from build123d import *

# Parameters (mm, degrees)
F0_R     = 11.25
F0_R_2   = 4.25
F1_DEPTH = 5.5
F2_SIZE2 = 6.25
F2_SIZE  = 1
F0_R_3   = 14
F3_DEPTH = 6
F4_SIZE  = 0.4


with BuildPart() as f1:
    # F0 (on Top) → F1 (new body)
    with BuildSketch(Plane.XY):
        Circle(F0_R)
        Circle(F0_R_2, mode=Mode.SUBTRACT)
    extrude(amount=F1_DEPTH)

    # F2
    f2_edges = [f1.edges().sort_by_distance(p)[0] for p in [
        (-4.25, 0, 5.5),
    ]]
    chamfer(f2_edges, length=F2_SIZE, length2=F2_SIZE2)

    # F0 (on Top) → F3 (join)
    with BuildSketch(Plane.XY):
        Circle(F0_R_3)
        Circle(F0_R, mode=Mode.SUBTRACT)
    extrude(amount=F3_DEPTH)

    # F4
    f4_edges = [f1.edges().sort_by_distance(p)[0] for p in [
        (-11.25, 0, 6),
    ]]
    chamfer(f4_edges, length=F4_SIZE)


solid = f1.part
Could you check a few things on this model? Use its own coordinates, in mm. Give positions to 0.01 mm unless a question says otherwise; leave off trailing zeros. Order: outer loops, then holes, each group sorted by start corner. A loop starts at its lowest first (then second) coordinate and runs counter-clockwise, first axis right, second up. Notation, with made-up numbers: (42, 41) - (55, 41) arc R27 cw to (55, 67) - close; hole circle Ø4 at (7.25, 18). An arc over 180 degrees is marked (long way). Return JSON: item names as keys, results as strings. Group by question number.
Q1. Please list where these lines run through material, in increasing order: line 1 along Y through (x, z) = (0, 2.95); line 2 along X through (y, z) = (2.5, 1.05); line 3 along X through (y, z) = (-1.5, 2.7). Write a range as [from, to].
Q2. Suppose I cut it at A-A, the plane x = 0. Please give me the cut outline in (y, z), and give its area (3 significant figures).
Q3. Will these pins go through, and if not, where does the flat tip stop? pin 1 Ø3 at (x, y) = (8, 8) entering from -Z; pin 2 Ø10 at (x, y) = (0, 0) entering from +Z; pin 3 Ø1.5 at (x, z) = (-8.5, 4) entering from -Y.
Q4. Suppose I cut it at C-C, the plane z = 2.45. Please give me the cut outline in (x, y).
Q5. Thinking about a two-plate mould opening in X: for faces 1 (the face through (12.932, -5.362, 2.958)), 2 (the face through (2.285, 3.584, 2.218)), 3 (the face through (-3.2, 11.5, 6)), which applies, pulls with the +X half, pulls with the -X half, needs draft (parallel to the pull), parting line crosses it, or undercut?
Resolved:
{
 "1": {"line 1": "y = [-14, -4.25], [4.25, 14]", "line 2": "x = [-13.77, -3.44], [3.44, 13.77]", "line 3": "x = [-13.92, -3.98], [3.98, 13.92]"},
 "2": {"outline": "(-14, 0) - (-4.25, 0) - (-4.25, 4.5) - (-10.5, 5.5) - (-11.25, 5.5) - (-11.25, 5.6) - (-11.65, 6) - (-14, 6) - close; (4.25, 0) - (14, 0) - (14, 6) - (11.65, 6) - (11.25, 5.6) - (11.25, 5.5) - (10.5, 5.5) - (4.25, 4.5) - close", "area": "104 mm2"},
 "3": {"pin 1": "stops at z = 0", "pin 2": "stops at z = 4.62", "pin 3": "stops at y = -11.66"},
 "4": {"outline": "circle Ø28 at (0, 0); hole circle Ø8.5 at (0, 0)"},
 "5": {"face 1": "parting line crosses it", "face 2": "undercut", "face 3": "needs draft"}
}
